Autodesk Fusion 360 part; units mm, degrees
sketch "Sketch1" plane through (0, 0, 0) normal (0, 0, 1) x (1, 0, 0)
  line L0 (0, 0) -> (0, -6)
  line L1 (0, -6) -> (75, -6)
  line L2 (75, -6) -> (128.0288, -31.8639)
  line L3 (128.0288, -31.8639) -> (130.6591, -26.4711)
  line L4 (0, 0) -> (76.3852, 0)
  line L5 (130.6591, -26.4711) -> (76.3852, 0)
  dimension "d9" = 6
  dimension "d10" = 75
  dimension "d11" = 59
  dimension "d12" = 154
  dimension "d13" = 6
extrude "Extrude1" add sketch "Sketch1" along normal blind 41
sketch "Sketch2" plane through (0, -6, 0) normal (0, -1, 0) x (1, 0, 0)
  line L0 (0, 0) -> (75, 0)
  line L1 (75, 0) -> (75, 41)
  line L2 (75, 41) -> (0, 41)
  line L3 (0, 41) -> (0, 0)
  circle A0 centre (27, 20.5) radius 7
  dimension "d16" = 14
  dimension "d17" = 27
  dimension "d18" = 20.5
extrude "Hole1" cut sketch "Sketch2" against normal blind 6 contours A0
sketch "Sketch3" plane through (12.0487, 24.7034, 0) normal (-0.4384, -0.8988, 0) x (0.8988, -0.4384, 0)
  line L0 (70.0398, 0) -> (129.0398, 0)
  line L1 (129.0398, 0) -> (129.0398, 41)
  line L2 (129.0398, 41) -> (70.0398, 41)
  line L3 (70.0398, 41) -> (70.0398, 0)
  circle A0 centre (102.0398, 20.5) radius 7
  dimension "d21" = 14
  dimension "d22" = 27
  dimension "d28" = 20.5
extrude "Hole2" cut sketch "Sketch3" against normal through all contours A0
fillet "Fillet1" radius 6 1 edges at (75, -6, 20.5)
fillet "Fillet1" radius 12 1 edges at (76.3852, 0, 20.5)
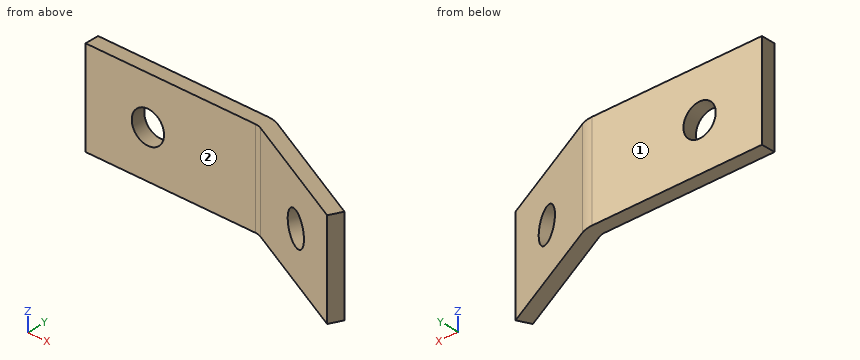
Read the model definition and answer for the solid it produces. Units are mm, in the model's axes. Face numbers are marked on the shaded views. A direction names the side the tool comes from. Coordinates: 2 decimals unless noted, no trailing zeros. Write each loop counter-clockwise with the first axis right and the second up, starting at its lowest first coordinate (ties: lowest second). Pieces come first, ordered by that corner, then holes. Notation, with made-up numbers: M 34.25,3.25 L 58.25,3.25 A16 cw 58.25,33.25 Z; hole C 76,-7 d2. An arc over 180 degrees is marked long. Use a Markdown table: item, result.
Q1. The part is cut by section C-C, the plane z = 35. Write down the section's boundary in (x, y).
Answer block:
| item | result |
|---|---|
| outline | M 0,-6 L 73.61,-6 A6 cw 76.25,-6.61 L 128.03,-31.86 L 130.66,-26.47 L 78.88,-1.21 A12 ccw 73.61,0 L 0,0 Z |
Q2. Which of the six approach directions +Z, -Z, +X, -X, +Y, -Y give full straight-line access (tool end or side, diameter ignored) to the marked faces 1 and 2?
Answer block:
| item | result |
|---|---|
| face 1 | +Z, -Z, +X, -X, +Y |
| face 2 | +Z, -Z, -X, -Y |
Q3. The part is cut by section A-A, the plane x = 27. Write down the section's boundary in (y, z).
Answer block:
| item | result |
|---|---|
| outline | M -6,0 L 0,0 L 0,13.5 L -6,13.5 Z; M -6,27.5 L 0,27.5 L 0,41 L -6,41 Z |
Q4. The part is cut by section D-D, the plane x = 12. Write down the section's boundary in (y, z), then the cut area to 3 significant figures.
Answer block:
| item | result |
|---|---|
| outline | M -6,0 L 0,0 L 0,41 L -6,41 Z |
| area | 246 mm2 |
Q5. Each of these flat-tipped pins is pushed along its axis until it touches: pin 1 Ø2 at (x, z) = (110.5, 35.5) entering from +Y; pin 2 Ø1 at (y, z) = (-24, 21.5) entering from +X; pin 3 Ø12.5 at (x, z) = (27, 20.5) entering from +Y; pin 4 Ø8 at (y, z) = (-13.5, 13.5) entering from -X. Where does it stop, or does it pass through?
Answer block:
| item | result |
|---|---|
| pin 1 | stops at y = -16.15 |
| pin 2 | stops at x = 126.62 |
| pin 3 | passes through |
| pin 4 | stops at x = 82.18 |
Q6. Straight lines are drawn through the part: L1, parallel to Z at x = 27, y = -2.4; L2, parallel to Y at x = 51, z = 27; L3, parallel to X at y = -4, z = 20. For each, find the intervals that lie inside material, in ascending order. Write a range as [from, to].
Answer block:
| item | result |
|---|---|
| L1 | z = [0, 13.5], [27.5, 41] |
| L2 | y = [-6, 0] |
| L3 | x = [0, 20.02], [33.98, 84.59] |
Q7. The part is cut by section B-B, the plane z = 16. Write down the section's boundary in (x, y), then the cut area to 3 significant figures.
Answer block:
| item | result |
|---|---|
| outline | M 0,-6 L 21.64,-6 L 21.64,0 L 0,0 Z; M 32.36,-6 L 73.61,-6 A6 cw 76.25,-6.61 L 98.94,-17.68 L 101.57,-12.28 L 78.88,-1.21 A12 ccw 73.61,0 L 32.36,0 Z; M 108.58,-22.38 L 128.03,-31.86 L 130.66,-26.47 L 111.21,-16.99 Z |
| area | 683 mm2 |
